Here's how the part is built. I have some questions about the finished solid (model axes, mm). A direction names the side the tool comes from. Coordinates: 2 decimals unless noted, no trailing zeros. Write each loop counter-clockwise with the first axis right and the second up, starting at its lowest first coordinate (ties: lowest second). Pieces come first, ordered by that corner, then holes. Notation, with made-up numbers: (-25, 31) -> (32, 31) arc R37 ccw to (32, 70) -> close; hole circle Ø8 at (50.25, 16). An arc over 180 degrees is marked (long way). Answer in a Markdown table with one row per item. Add a question column.
from build123d import *

# Parameters (mm, degrees)
F0_W     = 8.112996
F0_H     = 8.656824
F1_DEPTH = 50.1
F2_R     = 1.353874
F3_DEPTH = 25
F4_R     = 0.945263
F5_DEPTH = 5.2


with BuildPart() as f1:
    # F0 (on Top) → F1 (new body)
    with BuildSketch(Plane.XY):
        with Locations((4.056498, -4.328412)):
            Rectangle(F0_W, F0_H)
    extrude(amount=F1_DEPTH)

    # F2 (on face) → F3 (cut)
    with BuildSketch(Plane.YZ.offset(8.112996)):
        with Locations((-3.613207, 6.657105)):
            Circle(F2_R)
    extrude(amount=-F3_DEPTH, mode=Mode.SUBTRACT)

    # F4 (on face) → F5 (join)
    with BuildSketch(Plane.XY.offset(50.1)):
        with Locations((3.843431, -3.864297)):
            Circle(F4_R)
    extrude(amount=F5_DEPTH)


solid = f1.part
Q1. If we mould it in two halves opening along Z, with no side actions, what happens to faces 1 (the cylindrical face through (4.113, -3.907, 5.335)), 2 (the flat face through (0, -4, 25)), 3 (the flat face through (4, -4, 55.3))? For each: pulls with the +Z half, pulls with the -Z half, needs draft (parallel to the pull), parting line crosses it, or undercut.
Q2. Imagine slicing it at A-A on z = 7.5. Please give me the cut outline in (x, y), plus the area to 3 significant figures.
Q3. For faces 4 (the flat face through (4, -8.657, 25)), 5 (the cylindrical face through (4.745, -3.58, 52.664)), which set-ups out of +Z, -Z, +X, -X, +Y, -Y let a thin tool reach every point of the face, with its end or its side?
Q4. Imagine slicing it at C-C on y = -7.5. Please give me the cut outline in (x, z), plus the area to 3 significant figures.
Q5. Imagine slicing it at B-B on x = 0.75. Please give me the cut outline in (y, z).
Q6. I'm going to push a flat-ended pin straight in: P1, Ø1, axis at x = 6.5, y = -3.5, coming from the +Z side. Where does the tip first touch, or does it pass through?
Q7. I need wall thicknesses on line 1 (Z direction, x = 5.75, y = -0.5); line 2 (Z direction, x = 2.5, y = -4.75); line 3 (Z direction, x = 7.5, y = -4.5). Which ranges of each line are inside material? Lowest first, please. Write a range as [from, to].
Result sheet:
| question | item | result |
|---|---|---|
| 1 | face 1 | undercut |
| 1 | face 2 | needs draft |
| 1 | face 3 | pulls with the +Z half |
| 2 | outline | (0, -8.66) -> (8.11, -8.66) -> (8.11, -4.67) -> (0, -4.67) -> close; (0, -2.55) -> (8.11, -2.55) -> (8.11, 0) -> (0, 0) -> close |
| 2 | area | 53.0 mm^2 |
| 3 | face 4 | +Z, -Z, +X, -X, -Y |
| 3 | face 5 | +Z |
| 4 | outline | (0, 0) -> (8.11, 0) -> (8.11, 50.1) -> (0, 50.1) -> close |
| 4 | area | 406 mm^2 |
| 5 | outline | (-8.66, 0) -> (0, 0) -> (0, 50.1) -> (-8.66, 50.1) -> close; hole circle Ø2.71 at (-3.61, 6.66) |
| 6 | P1 | stops at z = 50.1 |
| 7 | line 1 | z = [0, 50.1] |
| 7 | line 2 | z = [0, 5.92], [7.39, 50.1] |
| 7 | line 3 | z = [0, 5.63], [7.68, 50.1] |
